The listing builds one solid part. Answer for the finished solid, in the listing's coordinates (mm). A direction names the side the tool comes from. Give positions to 0.01 mm unless a question says otherwise; leave off trailing zeros. Order: outer loops, then holes, each group sorted by start corner. A loop starts at its lowest first (then second) coordinate and runs counter-clockwise, first axis right, second up. Notation, with made-up numbers: (63.5, -17.75) - (69.5, -17.75) arc R25 ccw to (69.5, 12.25) - close; hole circle Ø8 at (9.5, 81.25). An arc over 180 degrees is marked (long way). Write each question's results on one line, items separated by ' | '. Start each with the question number.
1. Flat-ended cylindrical pins translate along their axes: pin 1 (2.5 mm diameter, centred on y = 3.5, z = 34.5, fed in from -X); pin 2 (2.5 mm diameter, centred on y = 3.5, z = 37.5, fed in from +X); pin 3 (2.5 mm diameter, centred on x = 48.5, y = 2, fed in from +Z). Find the tip coordinate at first contact, or state that the pin passes through.
2. Determine the mould class of faces 4 (the face through (-1.252, 2.465, 115.677)), 5 (the face through (85, 2, -63)), 6 (the face through (47, 3, 35)) for opening direction Z: released by +Z, released by -Z, zero draft, split by the parting line, or undercut.
3. Find the intervals of material crossed by L1, parallel to X at y = 2.75, z = -60; L2, parallel to X at y = 3.6, z = 76; L3, parallel to X at y = 1.9, z = 9, in increasing order.
4. Section B-B (y = 2.25) is taken. State how many separate pieces and enclosed holes the cut face has, and give its area (3 significant figures).
5. Section D-D (x = -36.5) is taken. Give the vertices of the cut face in (y, z), and give its area (3 significant figures).
6. Section A-A (z = -78) is taken. Give the vertices of the cut face in (x, y).
7. Which of the six approach directions +Z, -Z, +X, -X, +Y, -Y give full straight-line access (tool end or side, diameter ignored) to faces 1 (the face through (7.5, 3, 30)), 2 (the face through (-85, 2, -64)), 3 (the face through (91, 2, -100))?
8. Section C-C (x = 40.5) is taken. Give the vertices of the cut face in (y, z).
from build123d import *

# Parameters (mm, degrees)
EXTRUDE_1_DEPTH     = 5
SKETCH_3_R          = 2.25
SKETCH_3_R_2        = 1.75
SKETCH_3_R_3        = 1.5
SKETCH_3_W          = 13.356765245
SKETCH_3_H          = 10.34072148
CUT_EXTRUDE_1_DEPTH = 5
SKETCH_4_R          = 10
SKETCH_4_W          = 6
SKETCH_4_H          = 18
SKETCH_4_H_2        = 13
SKETCH_4_W_2        = 25
CUT_EXTRUDE_2_DEPTH = 166.168840415


with BuildPart() as part:
    # 草图1 → 凸台-拉伸1 (new body)
    with BuildSketch(Plane(origin=(0, 0, 0), x_dir=(1, 0, 0), z_dir=(0, 1, 0))):
        with BuildLine():
            Line((-93.991667227, 100), (-88, 100))
            ThreePointArc((-88, 100), (-85.878679656, 99.121320344), (-85, 97))
            Line((-85, 97), (-85, -91.739643711))
            ThreePointArc((-85, -91.739643711), (0, -115.681923528), (85, -91.739643711))
            Line((85, -91.739643711), (85, 97))
            ThreePointArc((85, 97), (85.878679656, 99.121320344), (88, 100))
            Line((88, 100), (93.991667227, 100))
            ThreePointArc((93.991667227, 100), (95.895095209, 101.386027753), (95.160319181, 103.62303808))
            ThreePointArc((95.160319181, 103.62303808), (0, 134.318076472), (-95.160319181, 103.62303808))
            ThreePointArc((-95.160319181, 103.62303808), (-95.895095209, 101.386027753), (-93.991667227, 100))
        make_face()
    extrude(amount=EXTRUDE_1_DEPTH)

    # 草图3 → 切除-拉伸1 (cut)
    with BuildSketch(Plane(origin=(0, 5, 0), x_dir=(1, 0, 0), z_dir=(0, 1, 0))):
        with Locations(Location((15, -100, 0), (0, 0, 270))):
            Circle(SKETCH_3_R)
        with Locations(Location((-15, -100, 0), (0, 0, 270))):
            Circle(SKETCH_3_R)
        with Locations(Location((-15, -76, 0), (0, 0, 270))):
            Circle(SKETCH_3_R)
        with Locations(Location((15, -76, 0), (0, 0, 270))):
            Circle(SKETCH_3_R)
        with Locations(Location((-18.5, 60, 0), (0, 0, 270))):
            Circle(SKETCH_3_R_2)
        with Locations(Location((18.5, 60, 0), (0, 0, 270))):
            Circle(SKETCH_3_R_2)
        with Locations(Location((18.5, 23, 0), (0, 0, 270))):
            Circle(SKETCH_3_R_2)
        with Locations(Location((-18.5, 23, 0), (0, 0, 270))):
            Circle(SKETCH_3_R_2)
        with Locations(Location((-8.5, 90, 0), (0, 0, 270))):
            Circle(SKETCH_3_R_2)
        with Locations(Location((0, 90, 0), (0, 0, 270))):
            Circle(SKETCH_3_R_2)
        with Locations(Location((8.5, 90, 0), (0, 0, 270))):
            Circle(SKETCH_3_R_2)
        with Locations(Location((0, 125, 0), (0, 0, 270))):
            Circle(SKETCH_3_R_3)
        with Locations(Location((19.76, -10, 0), (0, 0, 270))):
            Circle(SKETCH_3_R_2)
        with Locations(Location((19.76, -58.26, 0), (0, 0, 270))):
            Circle(SKETCH_3_R_2)
        with Locations(Location((-31.04, -15.08, 0), (0, 0, 270))):
            Circle(SKETCH_3_R_2)
        with Locations(Location((-31.04, -43.02, 0), (0, 0, 270))):
            Circle(SKETCH_3_R_2)
        with Locations(Location((47.445472194, 117.485375441, 0), (0, 0, 270))):
            Circle(SKETCH_3_R_3)
        with Locations(Location((-47.445472194, 117.485375441, 0), (0, 0, 270))):
            Circle(SKETCH_3_R_3)
        with BuildLine():
            Line((-85, 20), (-80.4, 20))
            ThreePointArc((-80.4, 20), (-79.717157288, 19.717157288), (-80, 20.4))
            Line((-80, 20.4), (-80, 29.6))
            ThreePointArc((-80, 29.6), (-79.717157288, 30.282842712), (-80.4, 30))
            Line((-80.4, 30), (-85, 30))
            Line((-85, 30), (-85, 20))
        make_face()
        with BuildLine():
            Line((-61, 29.6), (-61, 20.4))
            ThreePointArc((-61, 20.4), (-61.282842712, 19.717157288), (-60.6, 20))
            Line((-60.6, 20), (-56.4, 20))
            ThreePointArc((-56.4, 20), (-55.717157288, 19.717157288), (-56, 20.4))
            Line((-56, 20.4), (-56, 29.6))
            ThreePointArc((-56, 29.6), (-55.717157288, 30.282842712), (-56.4, 30))
            Line((-56.4, 30), (-60.6, 30))
            ThreePointArc((-60.6, 30), (-61.282842712, 30.282842712), (-61, 29.6))
        make_face()
        with BuildLine():
            Line((61, 29.6), (61, 20.4))
            ThreePointArc((61, 20.4), (61.282842712, 19.717157288), (60.6, 20))
            Line((60.6, 20), (56.4, 20))
            ThreePointArc((56.4, 20), (55.717157288, 19.717157288), (56, 20.4))
            Line((56, 20.4), (56, 29.6))
            ThreePointArc((56, 29.6), (55.717157288, 30.282842712), (56.4, 30))
            Line((56.4, 30), (60.6, 30))
            ThreePointArc((60.6, 30), (61.282842712, 30.282842712), (61, 29.6))
        make_face()
        with BuildLine():
            Line((85, 30), (85, 20))
            Line((85, 20), (80.4, 20))
            ThreePointArc((80.4, 20), (79.717157288, 19.717157288), (80, 20.4))
            Line((80, 20.4), (80, 29.6))
            ThreePointArc((80, 29.6), (79.717157288, 30.282842712), (80.4, 30))
            Line((80.4, 30), (85, 30))
        make_face()
        with Locations((29.239040261, 79.304944158)):
            Rectangle(SKETCH_3_W, SKETCH_3_H)
    extrude(amount=-CUT_EXTRUDE_1_DEPTH, mode=Mode.SUBTRACT)

    # 草图4 → 切除-拉伸2 (cut, through all)
    with BuildSketch(Plane(origin=(0, 5, 0), x_dir=(1, 0, 0), z_dir=(0, 1, 0))):
        with Locations(Location((0, 0, 0), (0, 0, 270))):
            Circle(SKETCH_4_R)
        with Locations((50, -5)):
            Rectangle(SKETCH_4_W, SKETCH_4_H)
        with Locations((50, -35)):
            Rectangle(SKETCH_4_W, SKETCH_4_H_2)
        with Locations((-5, -30)):
            Rectangle(SKETCH_4_W_2, SKETCH_4_H_2)
    extrude(amount=-CUT_EXTRUDE_2_DEPTH, mode=Mode.SUBTRACT)


solid = part.part
Reported:
1) pin 1: x = -85 | pin 2: x = 85 | pin 3: z = 108.68
2) face 4: released by +Z | face 5: zero draft | face 6: undercut
3) L1: -85 to -20.25, -16.75 to 16.75, 20.25 to 85 | L2: -85 to -17.25, -12.75 to 12.75, 17.25 to 85 | L3: -85 to -4.36, 4.36 to 18.32, 21.2 to 47, 53 to 85
4) separate pieces: 1 | enclosed holes: 25 | area: 38,700 mm²
5) outline: (0, -130.18) - (5, -130.18) - (5, 111.54) - (0, 111.54) - close | area: 1,210 mm²
6) outline: (-85, 0) - (22.56, 0) - (22.56, 5) - (-85, 5) - close; (35.92, 0) - (85, 0) - (85, 5) - (35.92, 5) - close
7) face 1: +Y, -Y | face 2: +Z, -X, +Y, -Y | face 3: +Z, +X, +Y, -Y
8) outline: (0, -129.2) - (5, -129.2) - (5, 110.57) - (0, 110.57) - close
